Can you work these out from the model? Positions are in its coordinate system, mm. Face numbers are marked on the shaded views. A direction names the side the tool comes from. Coordinates: 2 decimals unless noted, no trailing zeros. Order: outer loops, then holes, each group sorted by start corner. A loop starts at its lowest first (then second) coordinate and runs counter-clockwise, first axis right, second up. Notation, with made-up numbers: (-22, -39.5) -> (30, -39.5) arc R27 ccw to (30, -13.5) -> close; hole circle Ø4 at (-25.75, -34). An arc over 180 degrees is marked (long way). Answer in a Markdown table with one row per item. Add a question column.
1. Imagine slicing it at D-D on y = -27.5. Write out the boundary of the cut face in (x, z), plus the area to 3 significant figures.
2. Imagine slicing it at C-C on z = 55.5. Write out the boundary of the cut face in (x, y), plus the area to 3 significant figures.
3. On a 3-axis mill with a long thin cutter (end or side, diameter ignored), from which of +Z, -Z, +X, -X, +Y, -Y can I reach the whole of each face in a straight line? I mean the marked faces 1 and 2. Say none if no direction works.
4. If I drill on line 1 along Y through (x, z) = (0, 54.2); line 2 along Y through (x, z) = (-4, 53.25); line 3 along X through (y, z) = (-16, 56.5), over which ranges is the centre line in solid material (lowest first)? Write a range as [from, to].
5. We'd pull the mould along X, two halves only. Please class the marked faces 3, 4 and 5: pulls with the +X half, pulls with the -X half, needs draft (parallel to the pull), parting line crosses it, or undercut.
6. Will these pins go through, and if not, where does the flat tip stop? pin 1 (3 mm diameter, centred on x = 2.5, z = 54, fed in from +Y); pin 2 (4 mm diameter, centred on x = -18.5, z = 57.5, fed in from -Y); pin 3 (6 mm diameter, centred on x = -8.5, y = -20, fed in from -Z); pin 4 (5 mm diameter, centred on x = 10, y = -39, fed in from -Z).
7. Imagine slicing it at A-A on x = 0. Write out the boundary of the cut face in (y, z), plus the area to 3 significant figures.
8. Imagine slicing it at B-B on y = -39. Write out the boundary of the cut face in (x, z).
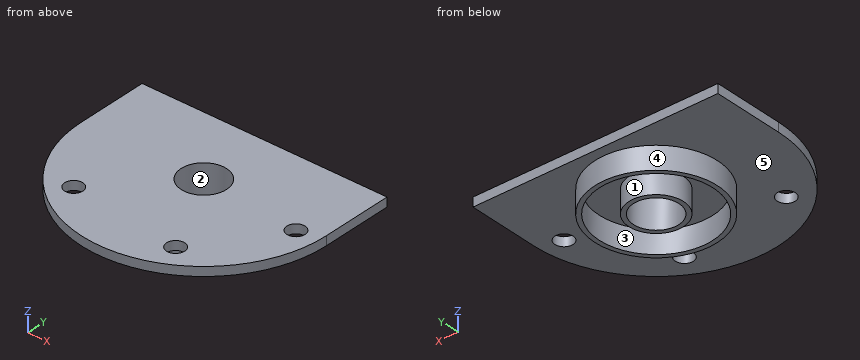
from build123d import *

# Parameters (mm, degrees)
CYLINDER003_R     = 5
CYLINDER003_DEPTH = 10
CYLINDER001_R     = 2
CYLINDER001_DEPTH = 10
CYLINDER002_R     = 2
CYLINDER002_DEPTH = 10
CYLINDER_R        = 2
CYLINDER_DEPTH    = 10
EXTRUDE005_DEPTH  = 2
SKETCH003_R       = 13.5
SKETCH003_R_2     = 12.5
SKETCH003_R_3     = 6
SKETCH003_R_4     = 5
EXTRUDE003_DEPTH  = 5


with BuildPart() as cylinder003:
    # Cylinder003 → Cylinder003 (new body)
    with BuildSketch(Plane(origin=(0, -20, 62), x_dir=(1, 0, 0), z_dir=(0, 0, -1))):
        Circle(CYLINDER003_R)
    extrude(amount=CYLINDER003_DEPTH)


with BuildPart() as cylinder001:
    # Cylinder001 → Cylinder001 (new body)
    with BuildSketch(Plane(origin=(10, -39, 55), x_dir=(1, 0, 0), z_dir=(0, 0, 1))):
        Circle(CYLINDER001_R)
    extrude(amount=CYLINDER001_DEPTH)


with BuildPart() as cylinder002:
    # Cylinder002 → Cylinder002 (new body)
    with BuildSketch(Plane(origin=(-15, -36, 54), x_dir=(1, 0, 0), z_dir=(0, 0, 1))):
        Circle(CYLINDER002_R)
    extrude(amount=CYLINDER002_DEPTH)


with BuildPart() as cylinder:
    # Cylinder → Cylinder (new body)
    with BuildSketch(Plane(origin=(22, -22, 54), x_dir=(1, 0, 0), z_dir=(0, 0, 1))):
        Circle(CYLINDER_R)
    extrude(amount=CYLINDER_DEPTH)


with BuildPart() as extrude005:
    # Sketch004 (on Face4 of Extrude003) → Extrude005 (new body)
    with BuildSketch(Plane.XY.offset(57)):
        with BuildLine():
            ThreePointArc((-26.964716, -20), (0, -46.964716), (26.964716, -20))
            Line((26.964716, -4.315231), (26.964716, -20))
            Line((-26.964716, -4.315231), (26.964716, -4.315231))
            Line((-26.964716, -20), (-26.964716, -4.315231))
        make_face()
    extrude(amount=EXTRUDE005_DEPTH)


with BuildPart() as cut003:
    # Sketch003 → Extrude003 (new body)
    with BuildSketch(Plane.XY.offset(52)):
        with Locations((0, -20)):
            Circle(SKETCH003_R)
        with Locations((0, -20)):
            Circle(SKETCH003_R_2, mode=Mode.SUBTRACT)
        with Locations((0, -20)):
            Circle(SKETCH003_R_3)
        with Locations((0, -20)):
            Circle(SKETCH003_R_4, mode=Mode.SUBTRACT)
    extrude(amount=EXTRUDE003_DEPTH)

    # Fusion: union Extrude005
    add(extrude005.part)

    # Cut: cut Cylinder
    add(cylinder.part, mode=Mode.SUBTRACT)

    # Cut001: cut Cylinder002
    add(cylinder002.part, mode=Mode.SUBTRACT)

    # Cut002: cut Cylinder001
    add(cylinder001.part, mode=Mode.SUBTRACT)

    # Cut003: cut Cylinder003
    add(cylinder003.part, mode=Mode.SUBTRACT)


solid = cut003.part
Answers follow:
| question | item | result |
|---|---|---|
| 1 | outline | (-25.9, 57) -> (-11.22, 57) -> (-11.22, 52) -> (-10, 52) -> (-10, 57) -> (10, 57) -> (10, 52) -> (11.22, 52) -> (11.22, 57) -> (25.9, 57) -> (25.9, 59) -> (-25.9, 59) -> close |
| 1 | area | 116 mm² |
| 2 | outline | circle Ø27 at (0, -20); circle Ø12 at (0, -20); hole circle Ø25 at (0, -20); hole circle Ø10 at (0, -20) |
| 2 | area | 116 mm² |
| 3 | face 1 | -Z |
| 3 | face 2 | +Z, -Z |
| 4 | line 1 | y = [-33.5, -32.5], [-26, -25], [-15, -14], [-7.5, -6.5] |
| 4 | line 2 | y = [-32.89, -31.84], [-24.47, -23], [-17, -15.53], [-8.16, -7.11] |
| 4 | line 3 | x = [-12.89, -11.84], [-4.47, -3], [3, 4.47], [11.84, 12.89] |
| 5 | face 3 | undercut |
| 5 | face 4 | parting line crosses it |
| 5 | face 5 | needs draft |
| 6 | pin 1 | stops at y = -6.54 |
| 6 | pin 2 | stops at y = -41.33 |
| 6 | pin 3 | stops at z = 52 |
| 6 | pin 4 | stops at z = 57 |
| 7 | outline | (-46.96, 57) -> (-33.5, 57) -> (-33.5, 52) -> (-32.5, 52) -> (-32.5, 57) -> (-26, 57) -> (-26, 52) -> (-25, 52) -> (-25, 59) -> (-46.96, 59) -> close; (-15, 52) -> (-14, 52) -> (-14, 57) -> (-7.5, 57) -> (-7.5, 52) -> (-6.5, 52) -> (-6.5, 57) -> (-4.32, 57) -> (-4.32, 59) -> (-15, 59) -> close |
| 7 | area | 85.3 mm² |
| 8 | outline | (-19.13, 57) -> (8, 57) -> (8, 59) -> (-19.13, 59) -> close; (12, 57) -> (19.13, 57) -> (19.13, 59) -> (12, 59) -> close |
